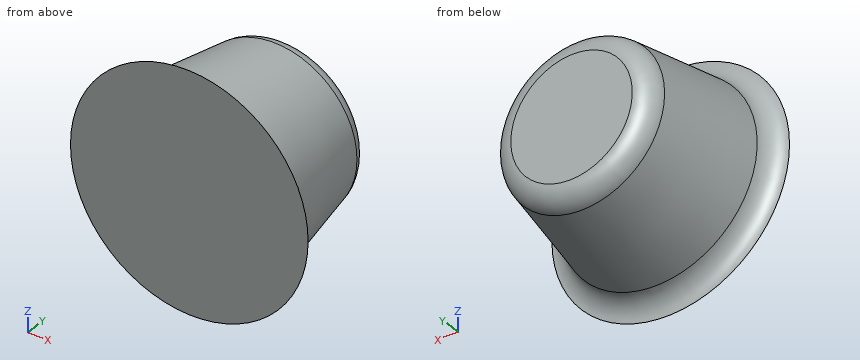
from build123d import *

# Parameters (mm, degrees)
SKETCH1_W           = 30
SKETCH1_H           = 30
BOSS_EXTRUDE1_DEPTH = 1
SKETCH2_R           = 7.5
BOSS_EXTRUDE2_DEPTH = 10
BOSS_EXTRUDE2_TAPER = 10
FILLET2_R           = 1.5


with BuildPart() as part:
    # Sketch1 → Boss-Extrude1 (new body)
    with BuildSketch(Plane(origin=(0, 0, 0), x_dir=(1, 0, 0), z_dir=(0, 1, 0))):
        Rectangle(SKETCH1_W, SKETCH1_H)
    extrude(amount=-BOSS_EXTRUDE1_DEPTH)

    # Sketch2 → Boss-Extrude2 (add)
    with BuildSketch(Plane(origin=(0, 0, 0), x_dir=(1, 0, 0), z_dir=(0, 1, 0))):
        Circle(SKETCH2_R)
    extrude(amount=BOSS_EXTRUDE2_DEPTH, taper=BOSS_EXTRUDE2_TAPER)

    # Fillet2
    fillet2_edges = [part.edges().sort_by_distance(p)[0] for p in [
        (-7.5, 0, 0),
        (-5.736730193, 10, 0),
    ]]
    fillet(fillet2_edges, radius=FILLET2_R)

    # SurfaceCut2
    split(bisect_by=Plane(origin=(0, 0, 0), x_dir=(1, 0, 0), z_dir=(0, 1, 0)), keep=Keep.TOP)


solid = part.part
Part model, mm, in its own coordinate system. Round coordinates to 2 decimals unless told otherwise and drop trailing zeros. Write each loop counter-clockwise with the first axis right and the second up, starting at its lowest first coordinate (ties: lowest second). Pieces come first, ordered by that corner, then holes. Notation, with made-up numbers: M 1,30.5 L 7,30.5 A21 ccw 7,40.5 Z; hole C 26,86 d6. An arc over 180 degrees is marked long. Return JSON: item names as keys, results as strings. Group by question number.
(1) Drill centre lines: probe 1 along Z at (x, y) = (4.5, 8); probe 2 along Z at (x, y) = (5.25, 1); probe 3 along X at (y, z) = (6.25, -5.75). Where is each one in solid material? Low to high.
(2) Pin check, flat tips, straight feed: pin 1 Ø1 at (x, y) = (0, 2) entering from -Z; pin 2 Ø4 at (y, z) = (2.5, 4.5) entering from -X; pin 3 Ø4 at (y, z) = (3, 6.5) entering from +X. Stop position of each tip, or through.
(3) Saw through at A-A on x = 0. Write the cut outline in (y, z), then the cut area to 3 significant figures.
Returned:
{
 "1": {"probe 1": "-4.1 to 4.1", "probe 2": "-5.14 to 5.14", "probe 3": "-2.81 to 2.81"},
 "2": {"pin 1": "z = -7.24", "pin 2": "x = -6.69", "pin 3": "x = 5.39"},
 "3": {"outline": "M 0,-8.76 A1.5 cw 1.24,-7.28 L 8.76,-5.96 A1.5 ccw 10,-4.48 L 10,4.48 A1.5 ccw 8.76,5.96 L 1.24,7.28 A1.5 cw 0,8.76 Z", "area": "132 mm²"}
}
